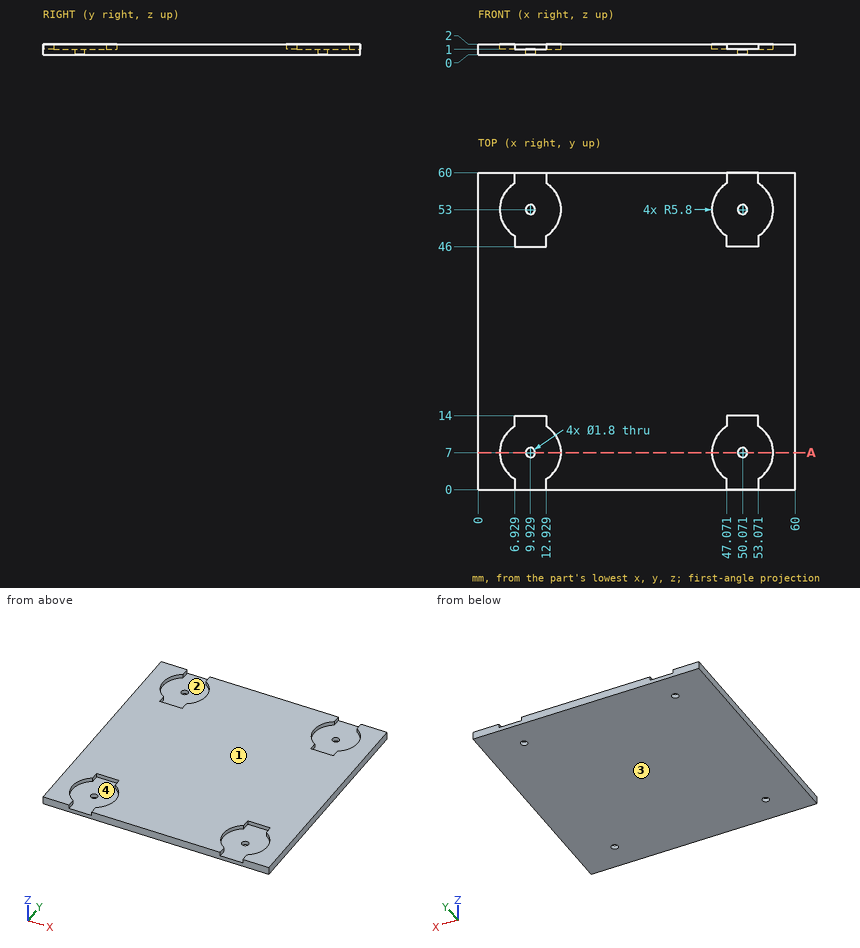
Design review of the part shown in the three views and the two pictorial views. Dimensions are in mm from the part's minimum x, y and z. A direction names the side the tool comes from. Round coordinates to 2 decimals unless told otherwise and drop trailing zeros. Write each loop counter-clockwise with the first axis right and the second up, starting at its lowest first coordinate (ties: lowest second). Pieces come first, ordered by that corner, then holes. Notation, with made-up numbers: (70, 2.25) -> (120, 2.25) arc R9 ccw to (120, 13.25) -> close; hole circle Ø2 at (71, 60.25). An arc over 180 degrees is marked (long way). Use one line per item in the form item = value.
1) Tool access review of the marked faces 1 and 2: name each direction out of +Z, -Z, +X, -X, +Y, -Y from which nothing blocks a thin tool from reaching the whole face with its end or side.
Found:
face_1 = +Z, +X, -X, +Y, -Y
face_2 = +Z
2) Clearance check with flat-ended pins moving along their axes: pin 1 (2 mm diameter, centred on x = 14.5, y = 12.5, fed in from -Z); pin 2 (0.5 mm diameter, centred on x = 51.5, z = 1.5, fed in from -Y); pin 3 (2 mm diameter, centred on x = 50.07, y = 7, fed in from +Z); pin 4 (0.8 mm diameter, centred on x = 9, z = 1.5, fed in from +Y). State where each tip first meets the part, or that it passes through.
Found:
pin_1 = 0
pin_2 = 14
pin_3 = 1
pin_4 = 46
3) Take a section at A-A, the plane y = 7. Write out the cut boundary in (x, z), and give its area (3 significant figures).
Found:
outline = (0, 0) -> (9.03, 0) -> (9.03, 1) -> (4.13, 1) -> (4.13, 2) -> (0, 2) -> close; (10.83, 0) -> (49.17, 0) -> (49.17, 1) -> (44.27, 1) -> (44.27, 2) -> (15.73, 2) -> (15.73, 1) -> (10.83, 1) -> close; (50.97, 0) -> (60, 0) -> (60, 2) -> (55.87, 2) -> (55.87, 1) -> (50.97, 1) -> close
area = 93.2 mm2
4) To check wall thickness, follow L1, parallel to X at y = 48, z = 1.75; L2, parallel to X at y = 7, z = 1.25; L3, parallel to Y at x = 10.5, z = 0.5. State the ranges of each line that lie inside material, in increasing order. Write a range as from..to.
Found:
L1 = 0..6.93, 12.93..47.07, 53.07..60
L2 = 0..4.13, 15.73..44.27, 55.87..60
L3 = 0..6.3, 7.7..52.3, 53.7..60
5) Mouldability with a two-part tool opening along Y and no side actions: class the marked faces 3 and 4 as +Y half, -Y half, draft (parallel to the pull), parting line (faces both ways), or undercut.
Found:
face_3 = draft
face_4 = undercut
